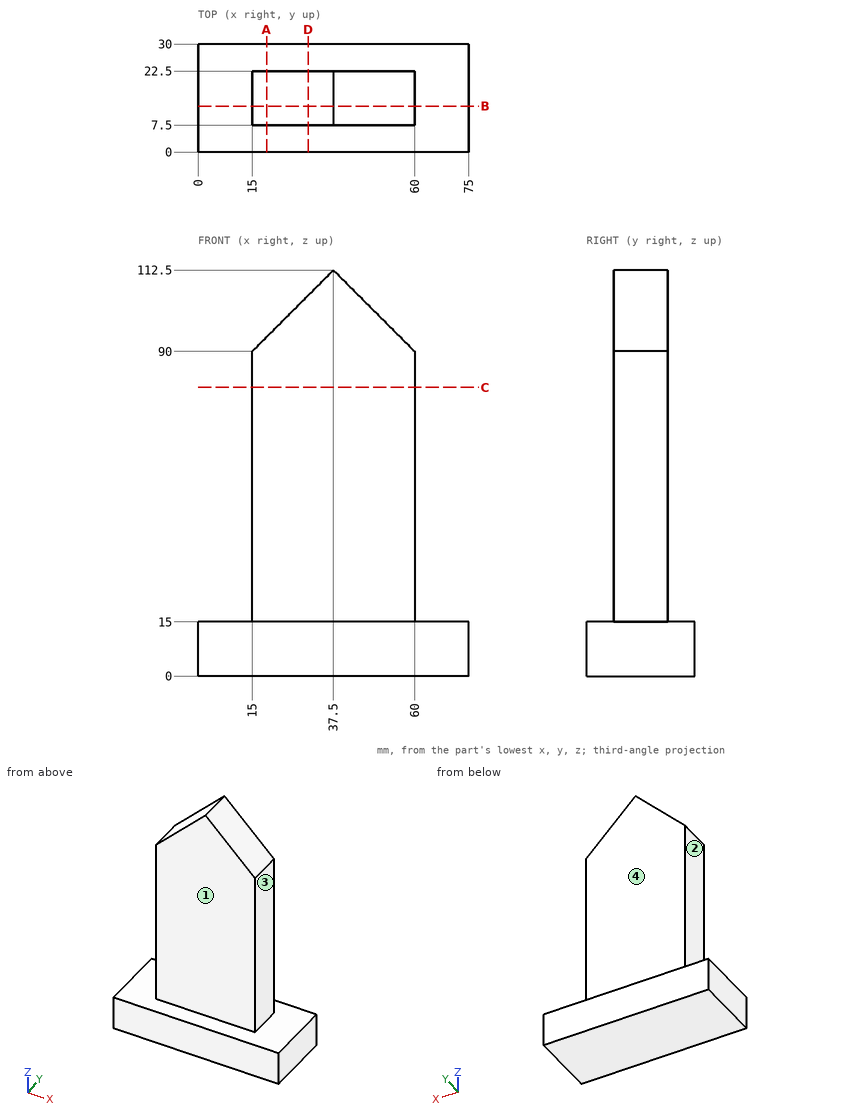
Can you work these out from the drawing? Everything is in mm from the part's minimum corner. A direction names the side the tool comes from. Give positions to 0.01 mm unless a question says otherwise; leave off trailing zeros. Order: outer loops, then holes, each group sorted by start corner. A loop starts at its lowest first (then second) coordinate and runs counter-clockwise, first axis right, second up.
1. I need wall thicknesses on L1, parallel to Z at x = 6.5, y = 3; L2, parallel to X at y = 15.5, z = 84; L3, parallel to Y at x = 57.5, z = 55. Which ranges of each line are inside material? Lowest first, please.
2. For the marked faces 1, 2, 3 and 4, which set-ups out of +Z, -Z, +X, -X, +Y, -Y let a thin tool reach every point of the face, with its end or its side?
3. Suppose I cut it at B-B (y = 12.75). List the corners of the cut face in (x, z) for me.
4. Suppose I cut it at C-C (z = 80). List the corners of the cut face in (x, y) for me, plus the area to 3 significant figures.
5. Suppose I cut it at A-A (x = 19). List the corners of the cut face in (y, z) for me.
6. Will these pins go through, and if not, where does the flat tip stop? P1, Ø12, axis at x = 45.5, z = 62.5, coming from the -Y side; P2, Ø16.5, axis at y = 13, z = 56, coming from the +X side; P3, Ø12, axis at x = 12, y = 15, coming from the +Z side.
7. Suppose I cut it at D-D (x = 30.5). List the corners of the cut face in (y, z) for me, plus the area to 3 significant figures.
Solved:
1. L1: z = 0 to 15
1. L2: x = 15 to 60
1. L3: y = 7.5 to 22.5
2. face 1: +Z, +X, -X, -Y
2. face 2: +Z, -X, +Y, -Y
2. face 3: +Z, +X, +Y, -Y
2. face 4: +Z, +X, -X, +Y
3. outline: (0, 0) - (75, 0) - (75, 15) - (60, 15) - (60, 90) - (37.5, 112.5) - (15, 90) - (15, 15) - (0, 15) - close
4. outline: (15, 7.5) - (60, 7.5) - (60, 22.5) - (15, 22.5) - close
4. area: 675 mm2
5. outline: (0, 0) - (30, 0) - (30, 15) - (22.5, 15) - (22.5, 94) - (7.5, 94) - (7.5, 15) - (0, 15) - close
6. P1: stops at y = 7.5
6. P2: stops at x = 60
6. P3: stops at z = 93
7. outline: (0, 0) - (30, 0) - (30, 15) - (22.5, 15) - (22.5, 105.5) - (7.5, 105.5) - (7.5, 15) - (0, 15) - close
7. area: 1,810 mm2
